```python
from build123d import *

# Parameters (mm, degrees)
F0_W          = 117.9976798594
F0_H          = 12.2914258391
F1_DEPTH      = 60
F4_DEPTH      = 10
F6_DEPTH      = 10
F7_W          = 39.3325621262
F7_H          = 90.9565519542
F8_DEPTH      = 57.5873161514
F8_DEPTH_BACK = 100
F9_R          = 2


with BuildPart() as f1:
    # F0 (on Front) → F1 (new body)
    with BuildSketch(Plane.XZ):
        with Locations((1.843707636, 29.4994218275)):
            Rectangle(F0_W, F0_H)
    extrude(amount=F1_DEPTH)

    # F3 (on offset) → F4 (join)
    with BuildSketch(Plane.XZ.offset(50)):
        Polygon((-28.8848504424, 23.353708908), (-40.7665632665, 23.7634219229), (-57.1551285684, -56.1308450997), (-42.4054190516, -56.1308450997), (-37.5268632135, -27.4508504777), (-35.645134747, -16.3885680959), align=None)
        Polygon((35.509279896, -16.3885680959), (-35.645134747, -16.3885680959), (-37.5268632135, -27.4508504777), (36.4408404675, -27.4508504777), align=None)
        Polygon((32.1625620127, 23.353708908), (35.509279896, -16.3885680959), (36.4408404675, -27.4508504777), (38.7179888785, -54.4919893146), (52.6482760906, -54.4919893146), (46.5025603771, 23.7634219229), align=None)
    extrude(amount=F4_DEPTH)

    # F5 (on Front) → F6 (join)
    with BuildSketch(Plane.XZ):
        Polygon((53.0579872429, -54.9017004669), (47.321986407, 24.1731368005), (33.1846513491, 23.4278501328), (36.0627619886, -16.2489450714), (36.7494194461, -25.7150048338), (36.9629519862, -28.6587022527), (38.9408726281, -55.9257402756), align=None)
        Polygon((36.7494194461, -25.7150048338), (36.0627619886, -16.2489450714), (-35.1216238776, -16.2489450714), (-36.8050870485, -25.7150048338), (36.9629519862, -28.6587022527), align=None)
        Polygon((-36.8050870485, -25.7150048338), (-35.1216238776, -16.2489450714), (-28.0654225498, 23.4278501328), (-41.1762744188, 23.4278501328), (-57.5863161514, -55.7236002397), (-41.9957078993, -54.9017004669), align=None)
    extrude(amount=F6_DEPTH)

    # F7 (on Right) → F8 (cut, two sides)
    with BuildSketch(Plane.YZ) as f8_sk:
        with Locations((-30.1139908843, -22.1245670691)):
            Rectangle(F7_W, F7_H)
    extrude(amount=-F8_DEPTH, mode=Mode.SUBTRACT)
    extrude(f8_sk.sketch, amount=F8_DEPTH_BACK, mode=Mode.SUBTRACT)

    # F9
    f9_edges = [f1.edges().sort_by_distance(p)[0] for p in [
        (1.843708, -60, 35.645135),
        (1.638856, -60, 23.353709),
        (-32.264993, -60, 3.48257),
        (33.835921, -60, 3.48257),
        (-0.067927, -60, -16.388568),
        (-0.543011, -60, -27.45085),
        (37.579415, -60, -40.97142),
        (49.591506, -60, -15.56914),
        (49.591506, -50, -15.56914),
        (60.842548, -30, 23.353709),
        (60.842548, -30, 35.645135),
        (1.843708, 0, 35.645135),
        (2.555711, 0, 23.353709),
        (54.111987, 0, 23.353709),
        (-57.155132, -30, 35.645135),
        (-57.155132, -30, 23.353709),
        (-57.155132, -60, 29.499422),
        (-57.155132, 0, 29.499422),
        (60.842548, 0, 29.499422),
        (60.842548, -60, 29.499422),
        (50.219707, 0, -15.773996),
        (-49.388981, 0, -16.184946),
        (-49.002868, -50, -16.388568),
        (-39.400397, 0, -40.308353),
        (-49.791012, 0, -55.31265),
        (0.078932, 0, -27.186854),
        (37.951912, 0, -42.292221),
        (45.99943, 0, -55.41372),
        (34.626396, 0, 3.552382),
        (0.470569, 0, -16.248945),
        (-31.600116, 0, 3.552382),
        (-31.600116, -10, 3.552382),
        (-39.400397, -10, -40.308353),
        (-39.966141, -60, -41.790848),
        (34.626396, -10, 3.552382),
        (50.219707, -10, -15.773996),
        (-49.002868, -60, -16.388568),
        (0.470569, -10, -16.248945),
        (-0.067927, -50, -16.388568),
        (-32.264993, -50, 3.48257),
        (-49.388981, -10, -16.184946),
        (-39.966141, -50, -41.790848),
        (37.951912, -10, -42.292221),
    ]]
    fillet(f9_edges, radius=F9_R)


solid = f1.part
```
Part model, mm, in its own coordinate system. A direction names the side the tool comes from. Give positions to 0.01 mm unless a question says otherwise; leave off trailing zeros. Write each loop counter-clockwise with the first axis right and the second up, starting at its lowest first coordinate (ties: lowest second). Pieces come first, ordered by that corner, then holes. Notation, with made-up numbers: (66.25, 26) -> (94.25, 26) arc R35 cw to (94.25, 59) -> close; hole circle Ø10 at (-21.5, -4.5). An arc over 180 degrees is marked (long way). Put each result on its own line as item: value. Start each with the question number.
Item 1: Cut at B-B (x = 9). State how many separate pieces and enclosed holes the cut face has, then the cut area to 3 significant figures.
Item 2: Wall check: L1, parallel to Y at x = 38, z = -15; L2, parallel to Z at x = 2, y = -23; L3, parallel to X at y = -7.5, z = 25. Give the ranges that are in metal, low to high. Write a range as [from, to].
Item 3: Pull direction Y, two halves, no side cores. Call faces 1 (the face through (2, -60, -21)), 2 (the face through (-40, -55, -42)), 3 (the face through (35.3, -9.4, 2.2)), 4 (the face through (-48.9, -9.4, -16.65)): pulls with the +Y half, pulls with the -Y half, needs draft (parallel to the pull), parting line crosses it, or undercut.
Item 4: Cut at A-A (y = -23). List the corners of the cut face in (x, z), then the cut area to 3 significant figures.
Item 5: Which spindle directions (+Z, -Z, +X, -X, +Y, -Y) get a long thin tool onto all of the face, cutting with end or side? Do faces 5 (the face through (37.938, -4.958, -42.101)), 6 (the face through (34.606, -4.958, 3.83)), 7 (the face through (-32.832, -59.399, 3.549)), 8 (the face through (49.53, -0.6, -14.18)), 9 (the face through (-31.65, -4.96, 3.28)). Say none if no direction does.
Item 6: Pin check, flat tips, straight feed: pin 1 Ø6.5 at (x, y) = (11, -53.5) entering from -Z; pin 2 Ø4 at (y, z) = (-27, 29) entering from -X; pin 3 Ø11 at (x, y) = (44, -53) entering from -Z. Stop position of each tip, or through.
Answer list:
1. separate pieces: 3
1. enclosed holes: 0
1. area: 952 mm2
2. L1: y = [-60, -50], [-10, 0]
2. L2: z = [23.35, 35.65]
2. L3: x = [-57.12, 60.81]
3. face 1: pulls with the -Y half
3. face 2: needs draft
3. face 3: undercut
3. face 4: undercut
4. outline: (-57.16, 25.35) arc R2 ccw to (-55.16, 23.35) -> (58.84, 23.35) arc R2 ccw to (60.84, 25.35) -> (60.84, 33.65) arc R2 ccw to (58.84, 35.65) -> (-55.16, 35.65) arc R2 ccw to (-57.16, 33.65) -> close
4. area: 1,450 mm2
5. face 5: -Z, +Y
5. face 6: +Y
5. face 7: -Y
5. face 8: +X, +Y
5. face 9: +Y, -Y
6. pin 1: stops at z = -27.45
6. pin 2: stops at x = -57.16
6. pin 3: stops at z = -54.49
